Could you check a few things on this model? Use its own coordinates, in mm. Face numbers are marked on the shaded views. A direction names the side the tool comes from. Coordinates: 2 decimals unless noted, no trailing zeros. Loops run counter-clockwise (first coordinate to the right, second up) from the corner with the lowest first, then second, coordinate; pieces in that order, holes last.
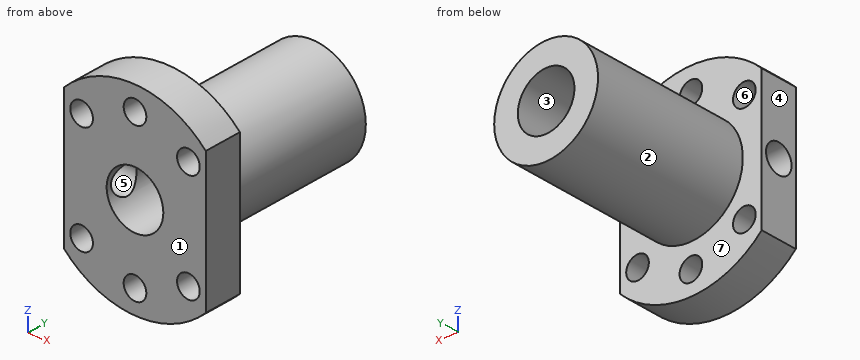
from build123d import *

# Parameters (mm, degrees)
SKETCH_1_R          = 2.4
SKETCH_1_R_2        = 11
EXTRUDE_1_DEPTH     = 8
SKETCH_1_3_R        = 11
SKETCH_1_3_R_2      = 6
EXTRUDE_2_DEPTH     = 42
SKETCH_2_R          = 3
CUT_EXTRUDE_1_DEPTH = 20


with BuildPart() as part:
    # Sketch 1 → Extrude 1 (new body)
    with BuildSketch(Plane(origin=(0, 0, 0), x_dir=(1, 0, 0), z_dir=(0, 1, 0))):
        with BuildLine():
            Line((15, 14.696938457), (15, -14.696938457))
            ThreePointArc((15, -14.696938457), (0, -21), (-15, -14.696938457))
            Line((-15, -14.696938457), (-15, 14.696938457))
            ThreePointArc((-15, 14.696938457), (0, 21), (15, 14.696938457))
        make_face()
        with Locations((0, 16)):
            Circle(SKETCH_1_R, mode=Mode.SUBTRACT)
        with Locations((11.313708499, 11.313708499)):
            Circle(SKETCH_1_R, mode=Mode.SUBTRACT)
        Circle(SKETCH_1_R_2, mode=Mode.SUBTRACT)
        with Locations((0, -16)):
            Circle(SKETCH_1_R, mode=Mode.SUBTRACT)
        with Locations((-11.313708499, -11.313708499)):
            Circle(SKETCH_1_R, mode=Mode.SUBTRACT)
        with Locations((11.313708499, -11.313708499)):
            Circle(SKETCH_1_R, mode=Mode.SUBTRACT)
        with Locations((-11.313708499, 11.313708499)):
            Circle(SKETCH_1_R, mode=Mode.SUBTRACT)
    extrude(amount=EXTRUDE_1_DEPTH)

    # Sketch 1_3 → Extrude 2 (add)
    with BuildSketch(Plane(origin=(0, 0, 0), x_dir=(1, 0, 0), z_dir=(0, 1, 0))):
        Circle(SKETCH_1_3_R)
        Circle(SKETCH_1_3_R_2, mode=Mode.SUBTRACT)
    extrude(amount=EXTRUDE_2_DEPTH)

    # Sketch 2 → Cut-Extrude 1 (cut)
    with BuildSketch(Plane.ZY.offset(15)):
        with Locations((0, 4)):
            Circle(SKETCH_2_R)
    extrude(amount=-CUT_EXTRUDE_1_DEPTH, mode=Mode.SUBTRACT)


solid = part.part
(1) Imagine slicing it at D-D, the plane z = 16. Write out the boundary of the cut face in (x, y), and give its area (3 significant figures).
Answers:
outline: (-13.6, 0) - (-2.4, 0) - (-2.4, 8) - (-13.6, 8) - close; (2.4, 0) - (13.6, 0) - (13.6, 8) - (2.4, 8) - close
area: 179 mm2
(2) Which directions (+Z, -Z, +X, -X, +Y, -Y) give clear straight access to the entire face, cutting with the end or side of a thin tool? Please do the marked faces 5, 6 and 7.
Answers:
face 5: -X
face 6: +Y, -Y
face 7: +Y
(3) We'd pull the mould along X, two halves only. Please class the marked faces 1, 2, 3 and 4: +X half, -X half, draft (parallel to the pull), parting line (faces both ways), or undercut.
Answers:
face 1: draft
face 2: parting line
face 3: undercut
face 4: -X half
(4) I need wall thicknesses on probe 1 along Y at (x, z) = (-9, 0); probe 2 along Y at (x, z) = (0.5, 12.5); probe 3 along X at (y, z) = (24, 0). Which ranges of each line are inside material? Lowest first, please.
Answers:
probe 1: y = 0 to 1, 7 to 42
probe 2: y = 0 to 8
probe 3: x = -11 to -6, 6 to 11
(5) For pin 1 (4 mm diameter, centred on x = -1.5, y = 38, fed in from -Z); pin 2 (3 mm diameter, centred on x = -9, y = 6, fed in from -Z); pin 3 (2 mm diameter, centred on x = 11, y = 30, fed in from +Z), each with a flat end and sliding along its axis, tell me the tip position at first contact or that it passes through.
Answers:
pin 1: stops at z = -11
pin 2: stops at z = -19.62
pin 3: stops at z = 4.58
(6) Imagine slicing it at A-A, the plane x = 0. Write out the boundary of the cut face in (y, z), and give its area (3 significant figures).
Answers:
outline: (0, -21) - (8, -21) - (8, -18.4) - (0, -18.4) - close; (0, -13.6) - (8, -13.6) - (8, -11) - (42, -11) - (42, -6) - (0, -6) - close; (0, 6) - (42, 6) - (42, 11) - (8, 11) - (8, 13.6) - (0, 13.6) - close; (0, 18.4) - (8, 18.4) - (8, 21) - (0, 21) - close
area: 503 mm2
(7) Imagine slicing it at B-B, the plane z = 0. Write out the boundary of the cut face in (x, y).
Answers:
outline: (-15, 0) - (-6, 0) - (-6, 1) - (-15, 1) - close; (-15, 7) - (-6, 7) - (-6, 42) - (-11, 42) - (-11, 8) - (-15, 8) - close; (6, 0) - (15, 0) - (15, 8) - (11, 8) - (11, 42) - (6, 42) - close
(8) Imagine slicing it at C-C, the plane y = 4. Write out the boundary of the cut face in (x, z).
Answers:
outline: (-15, -14.7) arc R21 ccw to (15, -14.7) - (15, 14.7) arc R21 ccw to (-15, 14.7) - (-15, 3) - (-5.2, 3) arc R6 cw (long way) to (-5.2, -3) - (-15, -3) - close; hole circle Ø4.8 at (-11.31, -11.31); hole circle Ø4.8 at (-11.31, 11.31); hole circle Ø4.8 at (0, -16); hole circle Ø4.8 at (0, 16); hole circle Ø4.8 at (11.31, -11.31); hole circle Ø4.8 at (11.31, 11.31)
